Read the model definition and answer for the solid it produces. Units are mm, in the model's axes. A direction names the side the tool comes from. Coordinates: 2 decimals unless noted, no trailing zeros. Loops run counter-clockwise (first coordinate to the right, second up) from the corner with the lowest first, then second, coordinate; pieces in that order, holes last. Notation, with made-up numbers: (-27, -22.5) -> (-12, -22.5) arc R18 cw to (-12, -13.5) -> close; hole circle Ø3 at (86, 19.5). An arc over 180 degrees is marked (long way). Answer as CSV lines item,"result".
```python
from build123d import *

# Parameters (mm, degrees)
CROQUIS1_R              = 2.5
SALIENTE_EXTRUIR1_DEPTH = 6
CROQUIS2_W              = 12.25
CROQUIS2_H              = 3.5
CORTAR_EXTRUIR1_DEPTH   = 7.5


with BuildPart() as part:
    # Croquis1 → Saliente-Extruir1 (new body)
    with BuildSketch(Plane(origin=(0, 0, 0), x_dir=(1, 0, 0), z_dir=(0, 1, 0))):
        with BuildLine():
            Line((-3.75, 34), (-3.75, -34))
            ThreePointArc((-3.75, -34), (0, -37.75), (3.75, -34))
            Line((3.75, -34), (3.75, 34))
            ThreePointArc((3.75, 34), (0, 37.75), (-3.75, 34))
        make_face()
        with Locations((0, 34)):
            Circle(CROQUIS1_R, mode=Mode.SUBTRACT)
        with Locations((0, -34)):
            Circle(CROQUIS1_R, mode=Mode.SUBTRACT)
        Circle(CROQUIS1_R, mode=Mode.SUBTRACT)
    extrude(amount=SALIENTE_EXTRUIR1_DEPTH)

    # Croquis2 → Cortar-Extruir1 (cut, symmetric)
    with BuildSketch(Plane(origin=(0, 0, 0), x_dir=(0, 0, -1), z_dir=(1, 0, 0))):
        with Locations((-33.875, 3)):
            Rectangle(CROQUIS2_W, CROQUIS2_H)
        with Locations((33.875, 3)):
            Rectangle(CROQUIS2_W, CROQUIS2_H)
    extrude(amount=CORTAR_EXTRUIR1_DEPTH, both=True, mode=Mode.SUBTRACT)


solid = part.part
```
Q1. A cutting plane is placed at D-D, the plane z = 0. Write down the section's boundary in (x, y), and give its area (3 significant figures).
Results:
outline,"(-3.75, 0) -> (-2.5, 0) -> (-2.5, 6) -> (-3.75, 6) -> close; (2.5, 0) -> (3.75, 0) -> (3.75, 6) -> (2.5, 6) -> close"
area,"15.0 mm²"
Q2. For faces 4 (the face through (0, 1.25, 31)), 5 (the face through (3.75, 3, 0)), 6 (the face through (0, 4.75, -30)), determine the directions among +Z, -Z, +X, -X, +Y, -Y from which every point of the face is accessible in a straight line to the end or side of a thin tool.
Results:
face 4,"+Z, +X, -X"
face 5,"+Z, -Z, +X, +Y, -Y"
face 6,"-Z, +X, -X"
Q3. Given pin 1 Ø1.8 at (x, y) = (-1, 2.5) entering from -Z; pin 2 Ø2 at (x, y) = (-2.5, 5) entering from -Z, each flat-ended and moving along its own axis, determine where each tip first touches the part or whether it passes through.
Results:
pin 1,"stops at z = -27.75"
pin 2,"stops at z = -37.44"
Q4. For a pull along Y with two mould halves and no side action, classify faces 1 (the face through (0, 4.75, 31)), 2 (the face through (-3, 0, -1)), 3 (the face through (-0.54, 2.96, 2.44)) as pulls with the +Y half, pulls with the -Y half, needs draft (parallel to the pull), parting line crosses it, or undercut.
Results:
face 1,"undercut"
face 2,"pulls with the -Y half"
face 3,"needs draft"
Q5. Find the intervals of material crossed by probe 1 along Z at (x, y) = (0, 2.6); probe 2 along Z at (x, y) = (0, 0.75); probe 3 along Y at (x, z) = (3.25, 32.5), in increasing order. Write a range as [from, to].
Results:
probe 1,"z = [-27.75, -2.5], [2.5, 27.75]"
probe 2,"z = [-37.75, -36.5], [-31.5, -2.5], [2.5, 31.5], [36.5, 37.75]"
probe 3,"y = [0, 1.25], [4.75, 6]"
Q6. A cutting plane is placed at B-B, the plane x = 0. Give the number of separate pieces and of enclosed holes in the cut face, and give its area (3 significant figures).
Results:
separate pieces,"6"
enclosed holes,"0"
area,"328 mm²"
Q7. A cutting plane is placed at A-A, the plane z = -30. Write down the section's boundary in (x, y).
Results:
outline,"(-3.75, 0) -> (3.75, 0) -> (3.75, 1.25) -> (-3.75, 1.25) -> close; (-3.75, 4.75) -> (3.75, 4.75) -> (3.75, 6) -> (-3.75, 6) -> close"
Q8. A cutting plane is placed at C-C, the plane y = 2.3. Write down the section's boundary in (x, z), and give its area (3 significant figures).
Results:
outline,"(-3.75, -27.75) -> (3.75, -27.75) -> (3.75, 27.75) -> (-3.75, 27.75) -> close; hole circle Ø5 at (0, 0)"
area,"397 mm²"
